```python
from build123d import *

# Parameters (mm, degrees)
F0_W     = 118
F0_H     = 40
F0_R     = 1.75
F0_W_2   = 30
F0_H_2   = 32
F1_DEPTH = 3
F3_DEPTH = 53
F5_DEPTH = 4
F6_W     = 53
F6_H     = 38
F7_DEPTH = 3
F9_DEPTH = 3
F10_R    = 0.99999


# Not quite as in the source:
# - a fillet or chamfer is up to 0.001 mm smaller than in the source, because OpenCascade refuses the exact size


with BuildPart() as f1:
    # F0 (on Top) → F1 (new body)
    with BuildSketch(Plane.XY):
        Rectangle(F0_W, F0_H)
        with Locations((-49, -1)):
            Circle(F0_R, mode=Mode.SUBTRACT)
        with Locations((-31, -1)):
            Rectangle(F0_W_2, F0_H_2, mode=Mode.SUBTRACT)
        with Locations((-13, -1)):
            Circle(F0_R, mode=Mode.SUBTRACT)
        with BuildLine():
            ThreePointArc((8, -3), (5, 0), (8, 3))
            Line((8, 3), (48, 3))
            ThreePointArc((48, 3), (51, 0), (48, -3))
            Line((48, -3), (8, -3))
        make_face(mode=Mode.SUBTRACT)
    extrude(amount=F1_DEPTH)

    # F2 (on face) → F3 (join)
    with BuildSketch(Plane(origin=(0, 0, 0), x_dir=(1, 0, 0), z_dir=(0, 0, -1))):
        Polygon((-56, 20), (-59, 20), (-59, 17), (-59, -20), (-56, -20), (-56, 17), (-46, 17), (-16, 17), (-6, 17), (-6, -11), (-3, -11), (-3, 17), (56, 17), (56, -20), (59, -20), (59, 17), (59, 20), (56, 20), align=None)
    extrude(amount=F3_DEPTH)

    # F4 (on face) → F5 (cut)
    with BuildSketch(Plane.YZ.offset(59)):
        with BuildLine():
            Line((10, -5), (-5, -5))
            ThreePointArc((-5, -5), (-7, -7), (-5, -9))
            Line((-5, -9), (10, -9))
            ThreePointArc((10, -9), (12, -7), (10, -5))
        make_face()
        with BuildLine():
            Line((10, -15), (-5, -15))
            ThreePointArc((-5, -15), (-7, -17), (-5, -19))
            Line((-5, -19), (10, -19))
            ThreePointArc((10, -19), (12, -17), (10, -15))
        make_face()
    extrude(amount=-F5_DEPTH, mode=Mode.SUBTRACT)

    # F6 (on face) → F7 (cut)
    with BuildSketch(Plane.XZ.offset(20)):
        with Locations((27.5, -21)):
            Rectangle(F6_W, F6_H)
    extrude(amount=-F7_DEPTH, mode=Mode.SUBTRACT)

    # F8 (on face) → F9 (cut)
    with BuildSketch(Plane.YZ.offset(-3)):
        with BuildLine():
            Line((-17, -53), (11, -53))
            Line((11, -53), (11, -23))
            Line((11, -23), (11, -10))
            ThreePointArc((11, -10), (-4.8004605743, -12.6220849169), (-17, -23))
            Line((-17, -23), (-17, -53))
        make_face()
    extrude(amount=-F9_DEPTH, mode=Mode.SUBTRACT)

    # F10 (radius 1 in the source; OpenCascade refuses exactly that, so slightly less here)
    f10_edges = [f1.edges().sort_by_distance(p)[0] for p in [
        (26.5, -17, 0),
        (-11, -17, 0),
        (-51, -17, 0),
        (27.5, -17, -2),
        (54, -20, -21),
        (27.5, -20, -40),
        (1, -20, -21),
        (1, -17, -21),
        (54, -17, -21),
        (27.5, -17, -40),
        (-16, -1, 3),
        (-31, -17, 3),
        (-46, -1, 3),
        (-31, 15, 3),
        (-31, 15, 0),
        (-16, -1, 0),
        (-46, -1, 0),
        (27.5, -20, -2),
        (-16, 15, 1.5),
        (-46, 15, 1.5),
        (-46, -17, 1.5),
        (-16, -17, 1.5),
        (54, -18.5, -2),
        (54, -18.5, -40),
        (1, -18.5, -40),
        (1, -18.5, -2),
        (-3, -3, 0),
        (-4.5, 11, 0),
        (-6, -3, 0),
        (-6, -17, -11.5),
        (-3, -17, -11.5),
        (-4.5, 11, -10),
    ]]
    fillet(f10_edges, radius=F10_R)


solid = f1.part
```
Can you work these out from the model? Positions are in its coordinate system, mm. A direction names the side the tool comes from. Coordinates: 2 decimals unless noted, no trailing zeros. Order: outer loops, then holes, each group sorted by start corner. A loop starts at its lowest first (then second) coordinate and runs counter-clockwise, first axis right, second up. Notation, with made-up numbers: (83, 80) - (119, 80) arc R22 ccw to (119, 90) - close; hole circle Ø3 at (28, 30.5). An arc over 180 degrees is marked (long way). Answer in a Markdown table with one row per item.
1. For pin 1 (0.9 mm diameter, centred on x = -4.5, z = -5.5, fed in from +Y); pin 2 (5.5 mm diameter, centred on x = -49, y = -1, fed in from -Z), each with a flat end and sliding along its axis, tell me the tip position at first contact or that it passes through.
Reply:
| item | result |
|---|---|
| pin 1 | stops at y = 11 |
| pin 2 | stops at z = 0 |
2. For faces 1 (the cylindrical face through (5, 0, 1)), 2 (the cylindrical face through (58, 12, -7)), 3 (the flat face through (-6, -6, -7)), which set-ups out of +Z, -Z, +X, -X, +Y, -Y let a thin tool reach every point of the face, with its end or its side?
Reply:
| item | result |
|---|---|
| face 1 | +Z, -Z |
| face 2 | +X |
| face 3 | -Z, +Y |
3. If I drill on line 1 along X through (y, z) = (-6.5, -49); line 2 along Y through (x, z) = (-13, 2); line 3 along Z through (x, y) = (-28, 17.5), over which ranges is the centre line in solid material (lowest first)?
Reply:
| item | result |
|---|---|
| line 1 | x = -59 to -56, 56 to 59 |
| line 2 | y = -20 to -2.75, 0.75 to 20 |
| line 3 | z = 0 to 3 |
4. Suppose I cut it at C-C (z = -7). Please give me the cut outline in (x, y), and give its area (3 significant figures).
Reply:
| item | result |
|---|---|
| outline | (-59, -20) - (0, -20) arc R1 ccw to (1, -19) - (1, -18) arc R1 ccw to (0, -17) - (-2, -17) arc R1 cw to (-3, -16) - (-3, 11) - (-6, 11) - (-6, -16) arc R1 cw to (-7, -17) - (-56, -17) - (-56, 20) - (-59, 20) - close; (54, -19) arc R1 ccw to (55, -20) - (59, -20) - (59, -7) - (56, -7) - (56, -17) - (55, -17) arc R1 ccw to (54, -18) - close; (56, 12) - (59, 12) - (59, 20) - (56, 20) - close |
| area | 444 mm^2 |
5. If we mould it in two halves opening along Y, with no side actions, what happens to faces 4 (the flat face through (-5, 11, -5)), 5 (the flat face through (28, -3, 1)), 6 (the flat face through (-59, 0, -25))? For each: pulls with the +Y half, pulls with the -Y half, needs draft (parallel to the pull), parting line crosses it, or undercut.
Reply:
| item | result |
|---|---|
| face 4 | pulls with the +Y half |
| face 5 | undercut |
| face 6 | needs draft |
6. Suppose I cut it at B-B (x = 36). Give the number of separate pieces and of enclosed holes in the cut face, and give its area (3 significant figures).
Reply:
| item | result |
|---|---|
| separate pieces | 3 |
| enclosed holes | 0 |
| area | 146 mm^2 |
7. Suppose I cut it at A-A (z = -34.5). Please give me the cut outline in (x, y).
Reply:
| item | result |
|---|---|
| outline | (-59, -20) - (0, -20) arc R1 ccw to (1, -19) - (1, -18) arc R1 ccw to (0, -17) - (-56, -17) - (-56, 20) - (-59, 20) - close; (54, -19) arc R1 ccw to (55, -20) - (59, -20) - (59, 20) - (56, 20) - (56, -17) - (55, -17) arc R1 ccw to (54, -18) - close |
8. Suppose I cut it at D-D (x = -49). Please give me the cut outline in (y, z).
Reply:
| item | result |
|---|---|
| outline | (-20, -53) - (-17, -53) - (-17, -1) arc R1 cw to (-16, 0) - (-2.75, 0) - (-2.75, 3) - (-20, 3) - close; (0.75, 0) - (20, 0) - (20, 3) - (0.75, 3) - close |
